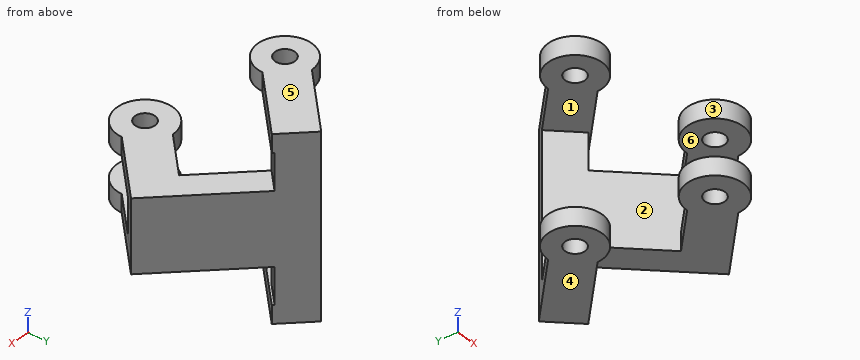
```python
from build123d import *

# Parameters (mm, degrees)
SKETCH1_R            = 7.75
SKETCH1_R_2          = 2.75
BOSS_EXTRUDE1_DEPTH  = 5
SKETCH2_R            = 7.75
SKETCH2_R_2          = 2.75
BOSS_EXTRUDE2_DEPTH  = 5
SKETCH3_R            = 7.5
SKETCH3_R_2          = 2.75
BOSS_EXTRUDE4_DEPTH  = 5
BOSS_EXTRUDE5_DEPTH  = 5
SKETCH6_W            = 20
SKETCH6_H            = 40.783378413
BOSS_EXTRUDE6_DEPTH  = 10
SKETCH7_R            = 2.75
CUT_EXTRUDE1_DEPTH   = 10
SKETCH9_R            = 2.75
CUT_EXTRUDE2_DEPTH   = 389.276117932
BOSS_EXTRUDE7_DEPTH  = 15
BOSS_EXTRUDE8_DEPTH  = 15
SKETCH12_R           = 7.5
SKETCH12_R_2         = 2.75
BOSS_EXTRUDE9_DEPTH  = 5
BOSS_EXTRUDE10_START = -5
SKETCH13_R           = 2.75
BOSS_EXTRUDE10_DEPTH = 5
CUT_EXTRUDE3_DEPTH   = 5
BOSS_EXTRUDE11_DEPTH = 2.5


with BuildPart() as part:
    # Sketch1 → Boss-Extrude1 (new body)
    with BuildSketch(Plane.XY):
        with Locations((-68.786796564, 328.786796564)):
            Circle(SKETCH1_R)
        with Locations((-68.786796564, 328.786796564)):
            Circle(SKETCH1_R_2, mode=Mode.SUBTRACT)
    extrude(amount=BOSS_EXTRUDE1_DEPTH)

    # Sketch4 → Boss-Extrude5 (add)
    with BuildSketch(Plane.XY):
        with BuildLine():
            Line((-61.036796564, 328.786796564), (-43.359127035, 346.464466094))
            Line((-43.359127035, 346.464466094), (-72.19733047, 375.30266953))
            Line((-72.19733047, 375.30266953), (-90, 357.5))
            ThreePointArc((-90, 357.5), (-95.303300859, 344.696699141), (-82.5, 350))
            Line((-82.5, 350), (-69.647077939, 362.852922061))
            Line((-69.647077939, 362.852922061), (-56.058874503, 349.264718626))
            Line((-56.058874503, 349.264718626), (-68.786796564, 336.536796564))
            ThreePointArc((-68.786796564, 336.536796564), (-74.266874119, 323.30671901), (-61.036796564, 328.786796564))
        make_face()
    extrude(amount=BOSS_EXTRUDE5_DEPTH)



with BuildPart() as body_2:
    # Sketch2 → Boss-Extrude2 (new body)
    with BuildSketch(Plane(origin=(0, 0, -10), x_dir=(-1, 0, 0), z_dir=(0, 0, -1))):
        with Locations((68.786796564, 328.786796564)):
            Circle(SKETCH2_R)
        with Locations((68.786796564, 328.786796564)):
            Circle(SKETCH2_R_2, mode=Mode.SUBTRACT)
    extrude(amount=BOSS_EXTRUDE2_DEPTH)

    # Sketch3 → Boss-Extrude4 (add)
    # profile 1 of 2: a face of its own
    with BuildSketch(Plane(origin=(0, 0, -15), x_dir=(-1, 0, 0), z_dir=(0, 0, -1))):
        with Locations((90, 350)):
            Circle(SKETCH3_R)
        with Locations((90, 350)):
            Circle(SKETCH3_R_2, mode=Mode.SUBTRACT)
    # profile 2 of 2: a face of its own
    with BuildSketch(Plane(origin=(0, 0, -15), x_dir=(-1, 0, 0), z_dir=(0, 0, -1))):
        with BuildLine():
            Line((43.359127035, 346.464466094), (61.036796564, 328.786796564))
            ThreePointArc((61.036796564, 328.786796564), (63.30671901, 334.266874119), (68.786796564, 336.536796564))
            Line((68.786796564, 336.536796564), (56.058874503, 349.264718626))
            Line((56.058874503, 349.264718626), (69.647077939, 362.852922061))
            Line((69.647077939, 362.852922061), (82.5, 350))
            ThreePointArc((82.5, 350), (84.696699141, 355.303300859), (90, 357.5))
            Line((90, 357.5), (72.19733047, 375.30266953))
            Line((72.19733047, 375.30266953), (43.359127035, 346.464466094))
        make_face()
    extrude(amount=-BOSS_EXTRUDE4_DEPTH)


with BuildPart() as part_1:
    add(part.part)

    add(body_2.part)  # Boss-Extrude6 merges body 2
    # Sketch6 → Boss-Extrude6 (add)
    with BuildSketch(Plane(origin=(151.55266953, 151.55266953, 0), x_dir=(0, 0, -1), z_dir=(0.7071067811865483, 0.7071067811865468, 0))):
        with Locations((5, 296.038595375)):
            Rectangle(SKETCH6_W, SKETCH6_H)
    extrude(amount=-BOSS_EXTRUDE6_DEPTH)

    # Sketch7 → Cut-Extrude1 (cut)
    with BuildSketch(Plane.XY.offset(5)):
        with Locations(Location((-68.786796564, 328.786796564, 0), (0, 0, 180))):
            Circle(SKETCH7_R)
        with Locations(Location((-90, 350, 0), (0, 0, 180))):
            Circle(SKETCH7_R)
    extrude(amount=-CUT_EXTRUDE1_DEPTH, mode=Mode.SUBTRACT)

    # Sketch9 → Cut-Extrude2 (cut, through all)
    with BuildSketch(Plane.XY.offset(5)):
        with BuildLine():
            Line((-82.5, 350), (-71.768398282, 360.731601718))
            Line((-71.768398282, 360.731601718), (-79.268398282, 368.231601718))
            Line((-79.268398282, 368.231601718), (-90, 357.5))
            ThreePointArc((-90, 357.5), (-95.303300859, 344.696699141), (-82.5, 350))
        make_face()
        with Locations((-90, 350)):
            Circle(SKETCH9_R, mode=Mode.SUBTRACT)
    extrude(amount=-CUT_EXTRUDE2_DEPTH, mode=Mode.SUBTRACT)

    # Sketch10 → Boss-Extrude7 (add)
    with BuildSketch(Plane.XY.offset(5)):
        Polygon((-72.19733047, 361.160533906), (-65.126262658, 368.231601718), (-72.19733047, 375.30266953), (-79.268398282, 368.231601718), align=None)
    extrude(amount=BOSS_EXTRUDE7_DEPTH)

    # Sketch11 → Boss-Extrude8 (add)
    with BuildSketch(Plane(origin=(0, 0, -15), x_dir=(-1, 0, 0), z_dir=(0, 0, -1))):
        Polygon((65.126262658, 368.231601718), (72.19733047, 361.160533906), (79.268398282, 368.231601718), (72.19733047, 375.30266953), align=None)
    extrude(amount=BOSS_EXTRUDE8_DEPTH)

    # Sketch12 → Boss-Extrude9 (add)
    # profile 1 of 3: a face of its own
    with BuildSketch(Plane.XY.offset(20)):
        with BuildLine():
            Line((-82.5, 350), (-71.768398282, 360.731601718))
            Line((-71.768398282, 360.731601718), (-72.19733047, 361.160533906))
            Line((-72.19733047, 361.160533906), (-79.268398282, 368.231601718))
            Line((-79.268398282, 368.231601718), (-90, 357.5))
            ThreePointArc((-90, 357.5), (-84.696699141, 355.303300859), (-82.5, 350))
        make_face()
    # profile 2 of 3: a face of its own
    with BuildSketch(Plane.XY.offset(20)):
        with Locations((-90, 350)):
            Circle(SKETCH12_R)
        with Locations((-90, 350)):
            Circle(SKETCH12_R_2, mode=Mode.SUBTRACT)
    # profile 3 of 3: a face of its own
    with BuildSketch(Plane.XY.offset(20)):
        Polygon((-72.19733047, 361.160533906), (-71.768398282, 360.731601718), (-64.69733047, 367.80266953), (-65.126262658, 368.231601718), align=None)
    extrude(amount=-BOSS_EXTRUDE9_DEPTH)

    # Sketch13 → Boss-Extrude10 (add)
    with BuildSketch(Plane(origin=(0, 0, -30), x_dir=(-1, 0, 0), z_dir=(0, 0, -1)).offset(BOSS_EXTRUDE10_START)):
        with BuildLine():
            Line((90, 357.5), (79.268398282, 368.231601718))
            Line((79.268398282, 368.231601718), (72.19733047, 361.160533906))
            Line((72.19733047, 361.160533906), (65.126262658, 368.231601718))
            Line((65.126262658, 368.231601718), (64.69733047, 367.80266953))
            Line((64.69733047, 367.80266953), (82.5, 350))
            ThreePointArc((82.5, 350), (95.303300859, 344.696699141), (90, 357.5))
        make_face()
        with Locations(Location((90, 350, 0), (0, 0, 180))):
            Circle(SKETCH13_R, mode=Mode.SUBTRACT)
    extrude(amount=BOSS_EXTRUDE10_DEPTH)

    # Sketch14 → Cut-Extrude3 (cut)
    with BuildSketch(Plane(origin=(151.55266953, 151.55266953, 0), x_dir=(0, 0, -1), z_dir=(0.7071067811865476, 0.7071067811865476, 0))):
        Polygon((-5, 275.646906168), (15, 275.646906168), (15, 306.430284581), (25, 306.430284581), (25, 305.823682863), (30, 305.823682863), (30, 316.430284581), (-20, 316.430284581), (-20, 305.823682863), (-15, 305.823682863), (-15, 306.430284581), (-5, 306.430284581), align=None)
    extrude(amount=-CUT_EXTRUDE3_DEPTH, mode=Mode.SUBTRACT)

    # Sketch15 → Boss-Extrude11 (add)
    with BuildSketch(Plane(origin=(148.017135624, 148.017135624, 0), x_dir=(0, 0, -1), z_dir=(0.7071067811865477, 0.7071067811865475, 0))):
        Polygon((-5, 306.430284581), (-5, 275.646906168), (15, 275.646906168), (15, 306.430284581), (25, 306.430284581), (25, 305.823682863), (30, 305.823682863), (30, 316.430284581), (-20, 316.430284581), (-20, 305.823682863), (-15, 305.823682863), (-15, 306.430284581), align=None)
    extrude(amount=BOSS_EXTRUDE11_DEPTH)


solid = part_1.part
```
The model under review builds one solid part; all positions refer to its coordinate system, in mm. Face numbers are marked on the shaded views. A direction names the side the tool comes from. Round coordinates to 2 decimals unless told otherwise and drop trailing zeros. Loops run counter-clockwise (first coordinate to the right, second up) from the corner with the lowest first, then second, coordinate; pieces in that order, holes last. Notation, with made-up numbers: (80, 33.5) -> (136, 33.5) arc R23 cw to (136, 53.5) -> close; hole circle Ø8 at (-24.75, 76.25). An arc over 180 degrees is marked (long way). Answer as a JSON object with one key per item and string values. Group by question number.
1) For the marked faces 5 and 6, list the 3-axis set-ups (+Z, -Z, +X, -X, +Y, -Y) from which the entire face can be reached by the end or side of a thin tool; tool diameter is ignored.
2) For pin 1 Ø12 at (y, z) = (356.5, 0) entering from -X; pin 2 Ø8 at (x, z) = (-55, 0) entering from -Y; pin 3 Ø6 at (x, z) = (-71.5, 9) entering from -Y, all flat-tipped, find the tip position at first contact; note any pin that passes through.
3) We need section A-A on x = -92. Write out the cut boundary in (y, z).
4) We need section D-D on z = -2. Write out the cut boundary in (x, y), then the cut area to 3 significant figures.
5) We need section C-C on y = 345.5. Write out the cut boundary in (x, z), then the cut area to 3 significant figures.
6) Mouldability with a two-part tool opening along Z and no side actions: class the marked faces 1, 2, 3 and 4 as released by +Z, released by -Z, zero draft, split by the parting line, or undercut.
7) We need section B-B on z = 4. Write out the cut boundary in (x, y).
8) For line 1 (X direction, y = 350, z = -26); line 2 (Z direction, x = -87, y = 346.5); line 3 (Y direction, x = -90, z = 18), list the stretches that pass through material, from the lowest coordinate up. Write a range as [from, to].
Result set:
{
 "1": {"face 5": "+Z, +X, -X, +Y, -Y", "face 6": "-X, -Y"},
 "2": {"pin 1": "x = -73.54", "pin 2": "y = 330.82", "pin 3": "y = 361.16"},
 "3": {"outline": "(342.77, -30) -> (348.11, -30) -> (348.11, -25) -> (342.77, -25) -> close; (342.77, 15) -> (348.11, 15) -> (348.11, 20) -> (342.77, 20) -> close; (351.89, -30) -> (357.23, -30) -> (357.23, -25) -> (351.89, -25) -> close; (351.89, 15) -> (357.23, 15) -> (357.23, 20) -> (351.89, 20) -> close"},
 "4": {"outline": "(-79.27, 368.23) -> (-50.43, 339.39) -> (-45.13, 344.7) -> (-73.97, 373.53) -> close", "area": "306 mm²"},
 "5": {"outline": "(-96, -30) -> (-84, -30) -> (-84, -25) -> (-96, -25) -> close; (-96, 15) -> (-84, 15) -> (-84, 20) -> (-96, 20) -> close; (-59.82, -15) -> (-45.93, -15) -> (-45.93, 5) -> (-59.82, 5) -> (-59.82, 0) -> (-56.54, 0) -> (-56.54, -10) -> (-59.82, -10) -> close", "area": "365 mm²"},
 "6": {"face 1": "undercut", "face 2": "undercut", "face 3": "zero draft", "face 4": "released by -Z"},
 "7": {"outline": "(-79.27, 368.23) -> (-58.18, 347.14) -> (-68.79, 336.54) arc R7.75 ccw (long way) to (-61.04, 328.79) -> (-45.13, 344.7) -> (-73.97, 373.53) -> close; hole circle Ø5.5 at (-68.79, 328.79)"},
 "8": {"line 1": "[-97.5, -92.75], [-87.25, -82.5]", "line 2": "[-30, -25], [15, 20]", "line 3": "[342.5, 347.25], [352.75, 357.5]"}
}
